from build123d import *

# Parameters (mm, degrees)
F0_R     = 9.5631
F1_DEPTH = 1.524
F3_DEPTH = 0.5
F4_R     = 4.04495
F5_DEPTH = 3.556
F6_R     = 0.7242640687
F7_SIZE2 = 1
F7_SIZE  = 0.5


with BuildPart() as f1:
    # F0 (on Top) → F1 (new body)
    with BuildSketch(Plane.XY):
        Circle(F0_R)
    extrude(amount=F1_DEPTH)

    # F2 (on face) → F3 (cut)
    with BuildSketch(Plane.XY.offset(1.524)):
        Polygon((8.7007693222, 0), (4.3503846611, 7.5350872655), (-4.3503846611, 7.5350872655), (-8.7007693222, 0), (-4.3503846611, -7.5350872655), (4.3503846611, -7.5350872655), align=None)
        Polygon((-7.7007693222, 0), (-3.8503846611, 6.6690618617), (3.8503846611, 6.6690618617), (7.7007693222, 0), (3.8503846611, -6.6690618617), (-3.8503846611, -6.6690618617), align=None, mode=Mode.SUBTRACT)
        Polygon((3.3503846611, 5.8030364579), (-3.3503846611, 5.8030364579), (-6.7007693222, 0), (-3.3503846611, -5.8030364579), (3.3503846611, -5.8030364579), (6.7007693222, 0), align=None)
        Polygon((-5.7007693222, 0), (-2.8503846611, 4.9370110541), (2.8503846611, 4.9370110541), (5.7007693222, 0), (2.8503846611, -4.9370110541), (-2.8503846611, -4.9370110541), align=None, mode=Mode.SUBTRACT)
        Polygon((2.3503846611, 4.0709856503), (-2.3503846611, 4.0709856503), (-4.7007693222, 0), (-2.3503846611, -4.0709856503), (2.3503846611, -4.0709856503), (4.7007693222, 0), align=None)
        Polygon((-3.7007693222, 0), (-1.8503846611, 3.2049602465), (1.8503846611, 3.2049602465), (3.7007693222, 0), (1.8503846611, -3.2049602465), (-1.8503846611, -3.2049602465), align=None, mode=Mode.SUBTRACT)
        Polygon((1.3503846611, 2.3389348427), (-1.3503846611, 2.3389348427), (-2.7007693222, 0), (-1.3503846611, -2.3389348427), (1.3503846611, -2.3389348427), (2.7007693222, 0), align=None)
        Polygon((-1.7007693222, 0), (-0.8503846611, 1.472909439), (0.8503846611, 1.472909439), (1.7007693222, 0), (0.8503846611, -1.472909439), (-0.8503846611, -1.472909439), align=None, mode=Mode.SUBTRACT)
    extrude(amount=-F3_DEPTH, mode=Mode.SUBTRACT)

    # F4 (on face) → F5 (join)
    with BuildSketch(Plane(origin=(0, 0, 0), x_dir=(1, 0, 0), z_dir=(0, 0, -1))):
        Circle(F4_R)
    extrude(amount=F5_DEPTH)

    # F6
    f6_edges = [f1.edges().sort_by_distance(p)[0] for p in [
        (-9.5631, 0, 0),
    ]]
    fillet(f6_edges, radius=F6_R)

    # F7
    f7_edges = [f1.edges().sort_by_distance(p)[0] for p in [
        (-4.04495, 0, -3.556),
    ]]
    f7_side = f1.faces().sort_by_distance((0, 0, -3.556))[0]
    chamfer(f7_edges, length=F7_SIZE, length2=F7_SIZE2, reference=f7_side)


solid = f1.part
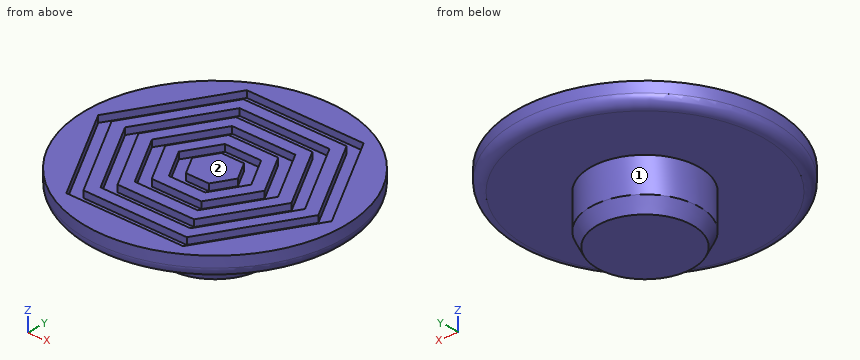
Work out the finished part from the listing and answer in its coordinate system (mm). Face numbers are marked on the shaded views. A direction names the side the tool comes from. Round coordinates to 2 decimals unless told otherwise and drop trailing zeros. Write each loop counter-clockwise with the first axis right and the second up, starting at its lowest first coordinate (ties: lowest second). Pieces come first, ordered by that corner, then holes. Notation, with made-up numbers: (60.25, 39) - (76.25, 39) arc R19 cw to (76.25, 55) - close; hole circle Ø10 at (73.25, 35). An arc over 180 degrees is marked (long way). Answer in a Markdown table with one row per item. Add a question column.
1. A cutting plane is placed at B-B, the plane z = -3.2. Determine the outline of the cut face in (x, y).
2. Find the intervals of material crossed by line 1 along Z through (x, y) = (1.75, 7.75); line 2 along Z through (x, y) = (-3, -5.25); line 3 along X through (y, z) = (-0.75, -1.95), in increasing order. Write a range as from..to.
3. Given pin 1 (1.5 mm diameter, centred on x = -5.5, y = -7, fed in from -Z), flat-ended and moving along its own axis, determine where the tip first touches the part or whether it passes through.
4. A cutting plane is placed at A-A, the plane z = -0.45. Determine the outline of the cut face in (x, y), and give its area (3 significant figures).
5. For the marked faces 1 and 2, determine the directions among +Z, -Z, +X, -X, +Y, -Y from which every point of the face is accessible in a straight line to the end or side of a thin tool.
Worked out:
| question | item | result |
|---|---|---|
| 1 | outline | circle Ø7.45 at (0, 0) |
| 2 | line 1 | 0..1.52 |
| 2 | line 2 | 0..1.02 |
| 2 | line 3 | -3.97..3.97 |
| 3 | pin 1 | z = 0 |
| 4 | outline | circle Ø8.09 at (0, 0) |
| 4 | area | 51.4 mm^2 |
| 5 | face 1 | -Z |
| 5 | face 2 | +Z, +X, -X, +Y, -Y |
